Autodesk Inventor part; units mm, degrees
ref_plane "Plano de trabajo1" through (190, 0, 0) normal (1, 0, 0) x (0, 0, -1)
ref_plane "YZ Plane" through (0, 0, 0) normal (1, 0, 0) x (0, 1, 0)
ref_plane "XZ Plane" through (0, 0, 0) normal (0, 1, 0) x (-1, 0, 0)
sketch "Boceto1" plane through (0, 0, 0) normal (1, 0, 0) x (0, 1, 0)
  circle A0 centre (0, 0) radius 60
  circle A1 centre (0, 0) radius 62
  line L0 (0, 0) -> (1013.9731, 0) construction
  dimension "d0" = 120
  dimension "d1" = 124
extrude "Extrusión1" add sketch "Boceto1" along normal blind 150
ref_plane "Plano de trabajo1" through (190, 0, 0) normal (1, 0, 0) x (0, 0, -1)
sketch "Boceto4" plane through (190, 0, 0) normal (1, 0, 0) x (0, 0, -1)
  circle A0 centre (0, 0) radius 30
  circle A1 centre (0, 0) radius 31.5
  dimension "d6" = 60
  dimension "d7" = 63
extrude "Extrusión2" add sketch "Boceto4" along normal blind 150
loft "Solevación1" add section 1 edges at (190, 0, 31.5) section 2 edges at (150, -62, 0) section 3 edges at (190, 0, 30)
properties part number "Tubo tolba" material "PVC, no plastificado"
Here's how the part is built. I have some questions about the finished solid (model axes, mm). A direction names the side the tool comes from. Round coordinates to 2 decimals unless told otherwise and drop trailing zeros. Order: outer loops, then holes, each group sorted by start corner. A loop starts at its lowest first (then second) coordinate and runs counter-clockwise, first axis right, second up. Notation, with made-up numbers: M 77,42 L 125,42 A30 cw 125,70 Z; hole C 13.5,26.5 d10. An arc over 180 degrees is marked long. One line per question, with ' | ' between items.
1) I want a section at A-A, the plane x = 99. Write out the boundary of the cut face in (y, z), then the cut area to 3 significant figures.
Working result:
outline: C 0,0 d124; hole C 0,0 d120 | area: 767 mm²
2) For pin 1 Ø10 at (x, y) = (303, -15.5) entering from +Z; pin 2 Ø4 at (x, z) = (56.5, -21.5) entering from -Y; pin 3 Ø1.5 at (x, z) = (53.5, -17) entering from -Y, each with a flat end and sliding along its axis, tell me the tip position at first contact or that it passes through.
Working result:
pin 1: z = 29.7 | pin 2: y = -58.85 | pin 3: y = -59.83
3) For faces 4 (the face through (73.95, -59.94, -2.64)), 5 (the face through (73.95, -8.071, -61.472)), which set-ups out of +Z, -Z, +X, -X, +Y, -Y let a thin tool reach every point of the face, with its end or its side?
Working result:
face 4: -X | face 5: +X, -X
4) I want a section at B-B, the plane x = 282. Write out the boundary of the cut face in (y, z), then the cut area to 3 significant figures.
Working result:
outline: C 0,0 d63; hole C 0,0 d60 | area: 290 mm²
5) If we mould it in two halves opening along Y, with no side actions, what happens to faces 1 (the face through (263.95, -31.232, 4.101)), 2 (the face through (340, -12, -28)), 3 (the face through (150, -51, 32))? For each: +Y half, -Y half, draft (parallel to the pull), parting line (faces both ways), or undercut.
Working result:
face 1: parting line | face 2: draft | face 3: undercut
6) I need wall thicknesses on line 1 along Y through (x, z) = (294, 0); line 2 along Y through (x, z) = (36.5, 2); line 3 along X through (y, z) = (-34, 51.5). Which ranges of each line are inside material? Lowest first, please.
Working result:
line 1: -31.5 to -30, 30 to 31.5 | line 2: -61.97 to -59.97, 59.97 to 61.97 | line 3: 0 to 150, 150.28 to 150.46
